Can you work these out from the drawing? Everything is in mm from the part's minimum corner. A direction names the side the tool comes from. Round coordinates to 2 decimals unless told otherwise and drop trailing zeros. Loops run counter-clockwise (first coordinate to the right, second up) from the corner with the lowest first, then second, coordinate; pieces in that order, holes last. Notation, with made-up numbers: M -30.75,6.25 L -1.75,6.25 A19 cw -1.75,26.25 Z; hole C 47,50.5 d10. An arc over 180 degrees is marked long. Answer in a Markdown table with one row per item.
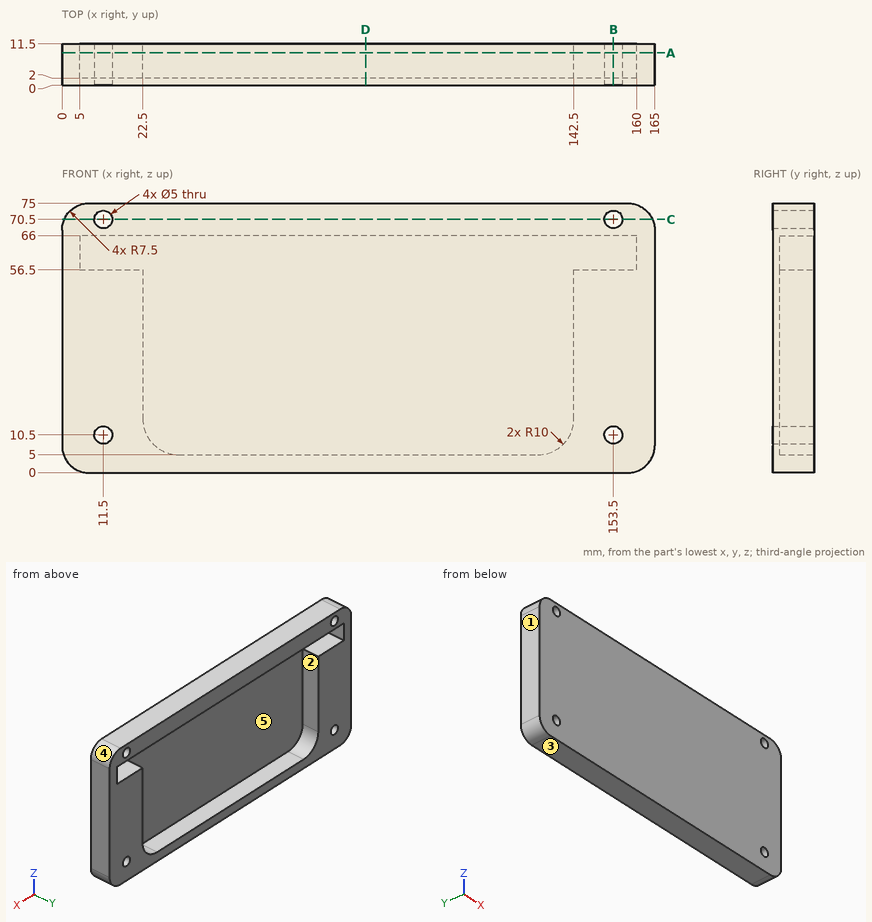
1) I want a section at C-C, the plane z = 70.5. Please give me the cut outline in (x, y), plus the area to 3 significant figures.
Computed:
| item | result |
|---|---|
| outline | M 0.63,0 L 9,0 L 9,11.5 L 0.63,11.5 Z; M 14,0 L 151,0 L 151,11.5 L 14,11.5 Z; M 156,0 L 164.37,0 L 164.37,11.5 L 156,11.5 Z |
| area | 1,770 mm² |
2) I want a section at D-D, the plane x = 84.5. Please give me the cut outline in (y, z), plus the area to 3 significant figures.
Computed:
| item | result |
|---|---|
| outline | M 0,0 L 11.5,0 L 11.5,5 L 2,5 L 2,66 L 11.5,66 L 11.5,75 L 0,75 Z |
| area | 283 mm² |
3) I want a section at A-A, the plane y = 9. Please give me the cut outline in (x, z).
Computed:
| item | result |
|---|---|
| outline | M 0,7.5 A7.5 ccw 7.5,0 L 157.5,0 A7.5 ccw 165,7.5 L 165,67.5 A7.5 ccw 157.5,75 L 7.5,75 A7.5 ccw 0,67.5 Z; hole M 5,56.5 L 22.5,56.5 L 22.5,15 A10 ccw 32.5,5 L 132.5,5 A10 ccw 142.5,15 L 142.5,56.5 L 160,56.5 L 160,66 L 5,66 Z; hole C 11.5,10.5 d5; hole C 11.5,70.5 d5; hole C 153.5,10.5 d5; hole C 153.5,70.5 d5 |
4) I want a section at B-B, the plane x = 153.5. Please give me the cut outline in (y, z), plus the area to 3 significant figures.
Computed:
| item | result |
|---|---|
| outline | M 0,0 L 11.5,0 L 11.5,8 L 0,8 Z; M 0,13 L 11.5,13 L 11.5,56.5 L 2,56.5 L 2,66 L 11.5,66 L 11.5,68 L 0,68 Z; M 0,73 L 11.5,73 L 11.5,75 L 0,75 Z |
| area | 657 mm² |
5) Which directions (+Z, -Z, +X, -X, +Y, -Y) give clear straight access to the entire face, cutting with the end or side of a thin tool? Please do the marked faces 1 and 2.
Computed:
| item | result |
|---|---|
| face 1 | +Z, -Z, -X, +Y, -Y |
| face 2 | +Y |
6) I need wall thicknesses on line 1 (Z direction, x = 153.5, y = 8.5); line 2 (X direction, y = 8, z = 29.5); line 3 (Z direction, x = 79.5, y = 7.75). Which ranges of each line are inside material? Lowest first, please.
Computed:
| item | result |
|---|---|
| line 1 | z = 0 to 8, 13 to 56.5, 66 to 68, 73 to 75 |
| line 2 | x = 0 to 22.5, 142.5 to 165 |
| line 3 | z = 0 to 5, 66 to 75 |
7) If we mould it in two halves opening along X, with no side actions, what happens to the marked faces 3, 4 and 5? For each: released by +X, released by -X, zero draft, split by the parting line, or undercut.
Computed:
| item | result |
|---|---|
| face 3 | zero draft |
| face 4 | released by +X |
| face 5 | undercut |
